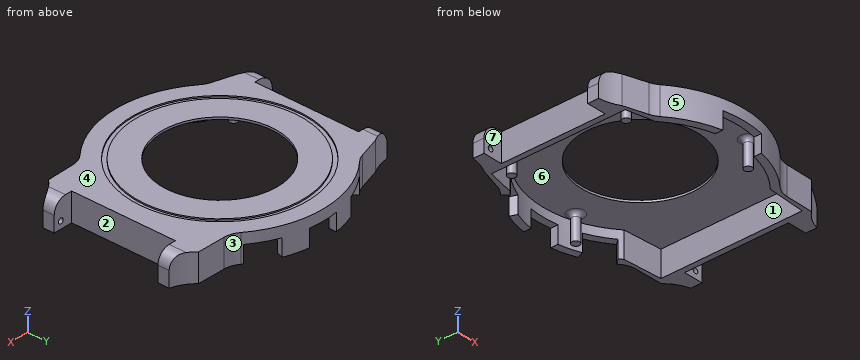
from build123d import *

# Parameters (mm, degrees)
PAD_DEPTH       = 6.5
POCKET_DEPTH    = 6
SKETCH002_R     = 13.5
POCKET001_DEPTH = 1
SKETCH003_W     = 5.4
SKETCH003_H     = 6.5
PAD001_DEPTH    = 4.5
POCKET002_DEPTH = 10
SKETCH008_R     = 0.6
POCKET003_DEPTH = 2
SKETCH009_R     = 0.6
POCKET004_DEPTH = 2
FILLET_R        = 2.9
FILLET001_R     = 2.9
FILLET002_R     = 5
FILLET003_R     = 5
FILLET004_R     = 5
FILLET005_R     = 5
SKETCH010_W     = 3.95
SKETCH010_H     = 6.5
PAD002_DEPTH    = 4.5
POCKET005_DEPTH = 10
SKETCH012_R     = 0.6
POCKET006_DEPTH = 2
SKETCH013_R     = 0.6
POCKET007_DEPTH = 2
FILLET006_R     = 3.4
FILLET007_R     = 3.4
SKETCH014_R     = 20.45
SKETCH014_R_2   = 19.5
POCKET008_DEPTH = 0.3
SKETCH015_R     = 0.9
PAD003_DEPTH    = 6
FILLET008_R     = 1
POCKET009_DEPTH = 4
POCKET010_DEPTH = 4


with BuildPart() as part:
    # Sketch → Pad (new body)
    with BuildSketch(Plane.XY):
        with BuildLine():
            Line((-22.5019915649, 16), (-22.5019915649, -16))
            Line((-22.5019915649, -16), (-16.2858834578, -17.9000000001))
            ThreePointArc((-16.2858834577, -17.9000000001), (0.2206895737, -24.1989937004), (16.6096357576, -17.5999999999))
            Line((16.6096357576, -17.6), (24.9082802252, -17.45))
            Line((24.9082802252, 17.45), (24.9082802252, -17.45))
            Line((16.6096357576, 17.6), (24.9082802252, 17.45))
            ThreePointArc((16.6096357576, 17.6), (0.2206895736, 24.1989937004), (-16.2858834578, 17.9))
            Line((-22.5019915649, 16), (-16.2858834578, 17.9))
        make_face()
    extrude(amount=PAD_DEPTH)

    # Sketch001 → Pocket (cut)
    with BuildSketch(Plane.XY):
        with BuildLine():
            Line((-14.8539557021, 16.9), (-21.2122180433, 15.55))
            Line((-21.2122180433, 15.55), (-21.2122180433, -15.55))
            Line((-21.2122180433, -15.55), (-14.8539557021, -16.9))
            ThreePointArc((-14.8539557021, -16.9), (-0.0760301383, -22.4998715423), (14.739402973, -17))
            Line((14.739402973, -17), (23.6191552218, -16.4))
            Line((23.6191552218, 16.4), (23.6191552218, -16.4))
            Line((14.739402973, 17), (23.6191552218, 16.4))
            ThreePointArc((14.739402973, 17), (-0.0760301383, 22.4998715423), (-14.8539557021, 16.9))
        make_face()
    extrude(amount=POCKET_DEPTH, mode=Mode.SUBTRACT)

    # Sketch002 (on Face19 of Pocket) → Pocket001 (cut)
    with BuildSketch(Plane(origin=(0, 0, 6), x_dir=(1, 0, 0), z_dir=(0, 0, -1))):
        Circle(SKETCH002_R)
    extrude(amount=-POCKET001_DEPTH, mode=Mode.SUBTRACT)

    # Sketch003 (on Face6 of Pocket001) → Pad001 (join)
    with BuildSketch(Plane.YZ.offset(24.9082802252)):
        with Locations((-14.75, 3.25)):
            Rectangle(SKETCH003_W, SKETCH003_H)
        with Locations((14.75, 3.25)):
            Rectangle(SKETCH003_W, SKETCH003_H)
    extrude(amount=PAD001_DEPTH)

    # Sketch006 → Pocket002 (cut)
    with BuildSketch(Plane.XY.offset(6.5)):
        with BuildLine():
            ThreePointArc((24.9082802253, 17.45), (26.9423471239, 15.7065020586), (29.4082802252, 14.6594169812))
            Line((29.4082802252, 17.45), (29.4082802252, 14.6594169812))
            Line((29.4082802252, 17.45), (24.9082802252, 17.45))
        make_face()
        with BuildLine():
            ThreePointArc((29.4082802253, -14.6594169812), (26.9423471239, -15.7065020586), (24.9082802253, -17.45))
            Line((29.4082802252, -17.45), (24.9082802252, -17.45))
            Line((29.4082802252, -14.6594169811), (29.4082802252, -17.45))
        make_face()
    extrude(amount=-POCKET002_DEPTH, mode=Mode.SUBTRACT)

    # Sketch008 (on Face27 of Pocket002) → Pocket003 (cut)
    with BuildSketch(Plane(origin=(0, -12.05, 0), x_dir=(-1, 0, 0), z_dir=(0, 1, 0))):
        with Locations((-27.7082802252, 1.7)):
            Circle(SKETCH008_R)
    extrude(amount=-POCKET003_DEPTH, mode=Mode.SUBTRACT)

    # Sketch009 (on Face26 of Pocket003) → Pocket004 (cut)
    with BuildSketch(Plane.XZ.offset(-12.05)):
        with Locations((27.7082802252, 1.7)):
            Circle(SKETCH009_R)
    extrude(amount=-POCKET004_DEPTH, mode=Mode.SUBTRACT)

    # Fillet
    fillet_edges = [part.edges().sort_by_distance(p)[0] for p in [
        (29.40828, -13.354708, 6.5),
    ]]
    fillet(fillet_edges, radius=FILLET_R)

    # Fillet001
    fillet001_edges = [part.edges().sort_by_distance(p)[0] for p in [
        (29.40828, 13.354708, 6.5),
    ]]
    fillet(fillet001_edges, radius=FILLET001_R)

    # Fillet002
    fillet002_edges = [part.edges().sort_by_distance(p)[0] for p in [
        (16.609636, -17.6, 3.25),
    ]]
    fillet(fillet002_edges, radius=FILLET002_R)

    # Fillet003
    fillet003_edges = [part.edges().sort_by_distance(p)[0] for p in [
        (16.609636, 17.6, 3.25),
    ]]
    fillet(fillet003_edges, radius=FILLET003_R)

    # Fillet004
    fillet004_edges = [part.edges().sort_by_distance(p)[0] for p in [
        (-16.285883, -17.9, 3.25),
    ]]
    fillet(fillet004_edges, radius=FILLET004_R)

    # Fillet005
    fillet005_edges = [part.edges().sort_by_distance(p)[0] for p in [
        (-16.285883, 17.9, 3.25),
    ]]
    fillet(fillet005_edges, radius=FILLET005_R)

    # Sketch010 (on Face4 of Fillet005) → Pad002 (join)
    with BuildSketch(Plane(origin=(-22.5019915649, 0, 0), x_dir=(0, -1, 0), z_dir=(-1, 0, 0))):
        with Locations((-14.025, 3.25)):
            Rectangle(SKETCH010_W, SKETCH010_H)
        with Locations((14.025, 3.25)):
            Rectangle(SKETCH010_W, SKETCH010_H)
    extrude(amount=PAD002_DEPTH)

    # Sketch011 (on Face6 of Pad002) → Pocket005 (cut)
    with BuildSketch(Plane.XY.offset(6.5)):
        with BuildLine():
            ThreePointArc((-27.0019915649, 14.6), (-24.6759937451, 15.0557212933), (-22.5019915649, 16))
            Line((-22.5019915649, 16), (-27.0019915649, 16))
            Line((-27.0019915649, 16), (-27.0019915649, 14.6))
        make_face()
        with BuildLine():
            ThreePointArc((-22.5019915649, -16), (-24.6759937451, -15.0557212933), (-27.0019915649, -14.6))
            Line((-27.0019915649, -14.6), (-27.0019915649, -16))
            Line((-27.0019915649, -16), (-22.5019915649, -16))
        make_face()
    extrude(amount=-POCKET005_DEPTH, mode=Mode.SUBTRACT)

    # Sketch012 (on Face23 of Pocket005) → Pocket006 (cut)
    with BuildSketch(Plane(origin=(0, -12.05, 0), x_dir=(-1, 0, 0), z_dir=(0, 1, 0))):
        with Locations((25.3019915649, 1.7)):
            Circle(SKETCH012_R)
    extrude(amount=-POCKET006_DEPTH, mode=Mode.SUBTRACT)

    # Sketch013 (on Face21 of Pocket006) → Pocket007 (cut)
    with BuildSketch(Plane.XZ.offset(-12.05)):
        with Locations((-25.3019915649, 1.7)):
            Circle(SKETCH013_R)
    extrude(amount=-POCKET007_DEPTH, mode=Mode.SUBTRACT)

    # Fillet006
    fillet006_edges = [part.edges().sort_by_distance(p)[0] for p in [
        (-27.001992, 13.325, 6.5),
    ]]
    fillet(fillet006_edges, radius=FILLET006_R)

    # Fillet007
    fillet007_edges = [part.edges().sort_by_distance(p)[0] for p in [
        (-27.001992, -13.325, 6.5),
    ]]
    fillet(fillet007_edges, radius=FILLET007_R)

    # Sketch014 (on Face4 of Fillet007) → Pocket008 (cut)
    with BuildSketch(Plane.XY.offset(6.5)):
        Circle(SKETCH014_R)
        Circle(SKETCH014_R_2, mode=Mode.SUBTRACT)
    extrude(amount=-POCKET008_DEPTH, mode=Mode.SUBTRACT)

    # Sketch015 (on Face55 of Pocket008) → Pad003 (join)
    with BuildSketch(Plane(origin=(0, 0, 6), x_dir=(1, 0, 0), z_dir=(0, 0, -1))):
        with Locations((-18.42, 13.32)):
            Circle(SKETCH015_R)
        with Locations((-18.42, -13.32)):
            Circle(SKETCH015_R)
        with Locations((7.27, 18.56)):
            Circle(SKETCH015_R)
        with Locations((5.37, -19.79)):
            Circle(SKETCH015_R)
    extrude(amount=PAD003_DEPTH)

    # Fillet008
    fillet008_edges = [part.edges().sort_by_distance(p)[0] for p in [
        (-19.32, -13.32, 6),
        (6.37, -18.56, 6),
        (-19.32, 13.32, 6),
        (4.47, 19.79, 6),
    ]]
    fillet(fillet008_edges, radius=FILLET008_R)

    # Sketch016 (on Face16 of Fillet008) → Pocket009 (cut)
    with BuildSketch(Plane(origin=(0, 0, 0), x_dir=(1, 0, 0), z_dir=(0, 0, -1))):
        with BuildLine():
            Line((-5, 23.6778377391), (-5, 21.9374109685))
            ThreePointArc((5, 21.9374109685), (0, 22.5), (-5, 21.9374109685))
            Line((5, 23.6778377391), (5, 21.9374109685))
            ThreePointArc((5, 23.6778377391), (0, 24.2), (-5, 23.6778377391))
        make_face()
    extrude(amount=-POCKET009_DEPTH, mode=Mode.SUBTRACT)

    # Sketch017 (on Face16 of Pocket009) → Pocket010 (cut)
    with BuildSketch(Plane(origin=(0, 0, 0), x_dir=(1, 0, 0), z_dir=(0, 0, -1))):
        with BuildLine():
            Line((-3.499984119, -22.2261132717), (-3.5, -23.9455632634))
            ThreePointArc((-3.5, -23.9455632634), (0, -24.2000019575), (3.5, -23.9455632634))
            Line((3.5000158811, -22.2261082701), (3.5, -23.9455632634))
            ThreePointArc((-3.499984119, -22.2261132717), (1.60767e-05, -22.5), (3.5000158811, -22.2261082701))
        make_face()
        with BuildLine():
            ThreePointArc((-13.9498796389, -17.6536358312), (-11.25, -19.4855715851), (-8.3135572795, -20.9077680626))
            Line((-8.3135572795, -20.9077680626), (-8.9416927184, -22.487466094))
            ThreePointArc((-15.0038705449, -18.987466094), (-12.1, -20.9578147716), (-8.9416927184, -22.487466094))
            Line((-13.9498796389, -17.6536358312), (-15.0038705449, -18.987466094))
        make_face()
        with BuildLine():
            ThreePointArc((8.3135572795, -20.9077680626), (11.25, -19.4855715851), (13.9498796389, -17.6536358312))
            Line((13.9498796389, -17.6536358312), (15.0038705449, -18.987466094))
            ThreePointArc((8.9416927184, -22.487466094), (12.1, -20.9578147716), (15.0038705449, -18.987466094))
            Line((8.3135572795, -20.9077680626), (8.9416927184, -22.487466094))
        make_face()
    extrude(amount=-POCKET010_DEPTH, mode=Mode.SUBTRACT)


solid = part.part
Could you check a few things on this model? Use its own coordinates, in mm. Face numbers are marked on the shaded views. A direction names the side the tool comes from. Give positions to 0.01 mm unless a question says otherwise; leave off trailing zeros. Order: outer loops, then holes, each group sorted by start corner. A loop starts at its lowest first (then second) coordinate and runs counter-clockwise, first axis right, second up.
Item 1: If we mould it in two halves opening along Y, with no side actions, what happens to the marked faces 1, 2, 3 and 4? For each: pulls with the +Y half, pulls with the -Y half, needs draft (parallel to the pull), parting line crosses it, or undercut.
Item 2: For the marked faces 5, 6 and 7, which set-ups out of +Z, -Z, +X, -X, +Y, -Y let a thin tool reach every point of the face, with its end or its side?
Item 3: I'm going to push flat-ended pins straight in: pin 1 (1.5 mm diameter, centred on x = 20.5, z = 1, fed in from -Y); pin 2 (1 mm diameter, centred on x = 28, z = 1.5, fed in from +Y); pin 3 (0.7 mm diameter, centred on x = 27.71, z = 1.7, fed in from -Y). Where does each tip first touch, or does it pass through?
Item 4: If we section it at A-A, the plane y = 8: Write out the boundary of the cut face in (x, z).
Item 5: I need wall thicknesses on line 1 (Y direction, x = 0, z = 6.35); line 2 (X direction, y = -10.5, z = 2); line 3 (Y direction, x = -3, z = 6.25). Which ranges of each line are inside material? Lowest first, please.
Item 6: If we section it at D-D, the plane x = -18.42: Write out the boundary of the cut face in (y, z).
Item 7: If we section it at C-C, the plane z = 1.7: Count the separate pieces of the cut face and the enclosed holes in it, plus the area to 3 significant figures.
Item 8: If we section it at B-B, the plane x = -2.5: Write out the boundary of the cut face in (y, z).
Values:
1. face 1: undercut
1. face 2: undercut
1. face 3: pulls with the +Y half
1. face 4: needs draft
2. face 5: +Z, -Z, -Y
2. face 6: -Z
2. face 7: +Z, -Z, -X
3. pin 1: stops at y = -17.54
3. pin 2: stops at y = 15.39
3. pin 3: stops at y = -15.46
4. outline: (-22.5, 0) - (-21.21, 0) - (-21.21, 6) - (-10.87, 6) - (-10.87, 6.5) - (-17.78, 6.5) - (-17.78, 6.2) - (-18.82, 6.2) - (-18.82, 6.5) - (-22.5, 6.5) - close; (10.87, 6) - (23.62, 6) - (23.62, 0) - (24.91, 0) - (24.91, 6.5) - (18.82, 6.5) - (18.82, 6.2) - (17.78, 6.2) - (17.78, 6.5) - (10.87, 6.5) - close
5. line 1: y = -24.2 to -20.45, -19.5 to -13.5, 13.5 to 19.5, 20.45 to 24.2
5. line 2: x = -22.5 to -21.21, 23.62 to 24.91
5. line 3: y = -24.01 to -20.23, -19.27 to -13.16, 13.16 to 19.27, 20.23 to 24.01
6. outline: (-17.25, 0) - (-16.14, 0) - (-16.14, 6) - (-15.22, 6) arc R1 cw to (-14.22, 5) - (-14.22, 0) - (-12.42, 0) - (-12.42, 5) arc R1 cw to (-11.42, 6) - (11.42, 6) arc R1 cw to (12.42, 5) - (12.42, 0) - (14.22, 0) - (14.22, 5) arc R1 cw to (15.22, 6) - (16.14, 6) - (16.14, 0) - (17.25, 0) - (17.25, 6.5) - (8.88, 6.5) - (8.88, 6.2) - (6.4, 6.2) - (6.4, 6.5) - (-6.4, 6.5) - (-6.4, 6.2) - (-8.88, 6.2) - (-8.88, 6.5) - (-17.25, 6.5) - close
7. separate pieces: 8
7. enclosed holes: 0
7. area: 240 mm2
8. outline: (-24.07, 4) - (-22.36, 4) - (-22.36, 6) - (-13.27, 6) - (-13.27, 6.5) - (-19.34, 6.5) - (-19.34, 6.2) - (-20.3, 6.2) - (-20.3, 6.5) - (-24.07, 6.5) - close; (13.27, 6) - (22.36, 6) - (22.36, 4) - (24.07, 4) - (24.07, 6.5) - (20.3, 6.5) - (20.3, 6.2) - (19.34, 6.2) - (19.34, 6.5) - (13.27, 6.5) - close
